Geometry: see drawing. Coordinates: mm, zero at the bounding-box minimum. Give positions to 0.01 mm unless a question says otherwise; leave off trailing zeros. Loops run counter-clockwise (first coordinate to the right, second up) from the corner with the lowest first, then second, coordinate; pieces in that order, holes last. Notation, with made-up numbers: (34, 7) -> (85, 7) arc R28 cw to (85, 32) -> close; hole circle Ø11 at (36.5, 4). An arc over 180 degrees is marked (long way). Return JSON: item names as keys, results as strings. Group by question number.
(1) Cut plane B-B on y = 48. Return loops of the section in (x, z), then the cut area to 3 significant figures.
(2) Cut plane A-A on y = 6. Return loops of the section in (x, z), then the cut area to 3 significant figures.
(3) Cut plane D-D on x = 62. Return loops of the section in (y, z).
(4) Ray query, line 1 (X direction, y = 6, z = 5); line 2 (X direction, y = 48, z = 4.5); line 3 (Y direction, x = 34, z = 9). Return the intervals inside material, ascending. Write a range as from..to.
(5) Cut plane C-C on z = 6.25. Return loops of the section in (x, y), then the cut area to 3 significant figures.
(6) Draft query along Y for the marked faces 1, 2 and 3. Return one class per face: released by +Y, released by -Y, zero draft, split by the parting line, or undercut.
(7) Pin query (flat end, axial travel): pin 1 (2 mm diameter, centred on y = 19.5, z = 8.5, fed in from -X); pin 2 (4.5 mm diameter, centred on x = 60, y = 6, fed in from -Z). Return the tip coordinate at first contact, or that it passes through.
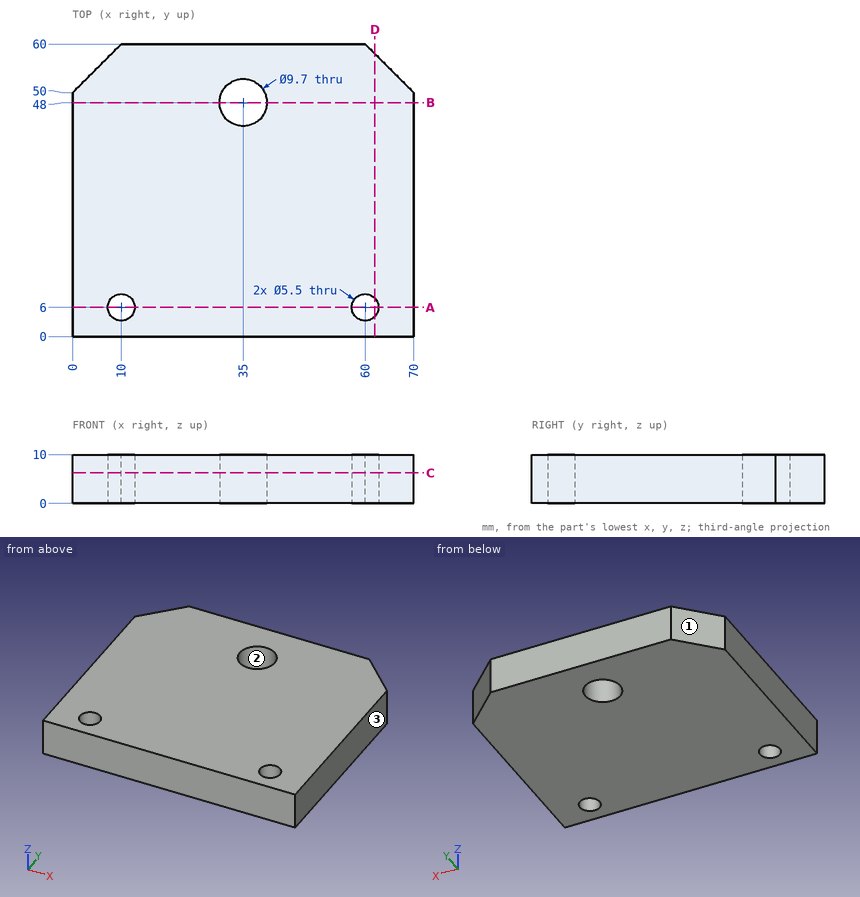
Answers:
{
 "1": {"outline": "(0, 0) -> (30.15, 0) -> (30.15, 10) -> (0, 10) -> close; (39.85, 0) -> (70, 0) -> (70, 10) -> (39.85, 10) -> close", "area": "603 mm²"},
 "2": {"outline": "(0, 0) -> (7.25, 0) -> (7.25, 10) -> (0, 10) -> close; (12.75, 0) -> (57.25, 0) -> (57.25, 10) -> (12.75, 10) -> close; (62.75, 0) -> (70, 0) -> (70, 10) -> (62.75, 10) -> close", "area": "590 mm²"},
 "3": {"outline": "(0, 0) -> (4.11, 0) -> (4.11, 10) -> (0, 10) -> close; (7.89, 0) -> (58, 0) -> (58, 10) -> (7.89, 10) -> close"},
 "4": {"line 1": "0..7.25, 12.75..57.25, 62.75..70", "line 2": "0..30.15, 39.85..70", "line 3": "0..43.25, 52.75..60"},
 "5": {"outline": "(0, 0) -> (70, 0) -> (70, 50) -> (60, 60) -> (10, 60) -> (0, 50) -> close; hole circle Ø5.5 at (10, 6); hole circle Ø9.7 at (35, 48); hole circle Ø5.5 at (60, 6)", "area": "3,980 mm²"},
 "6": {"face 1": "released by +Y", "face 2": "undercut", "face 3": "zero draft"},
 "7": {"pin 1": "x = 0", "pin 2": "through"}
}
